For this review, take the finished solid that the model builds, in its own axes (mm). A direction names the side the tool comes from. Coordinates: 2 decimals unless noted, no trailing zeros. Loops run counter-clockwise (first coordinate to the right, second up) from the corner with the lowest first, then second, coordinate; pieces in that order, holes last. Notation, with made-up numbers: (50, 64) - (97, 64) arc R24 cw to (97, 93) - close; hole circle Ø7 at (76.25, -24.5). An arc over 180 degrees is marked (long way). One line per item, written item: value. Start each with the question number.
1. Take a section at D-D, the plane y = 1. State the section outline as (x, z) points.
2. Take a section at C-C, the plane y = -9.5. State the section outline as (x, z) points.
3. For faces 1 (the face through (-45.514, 2, 2)), 2 (the face through (-8, -35.503, 2)), 3 (the face through (-23.58, 22.1, 1.67)), list the 3-axis set-ups (+Z, -Z, +X, -X, +Y, -Y) from which the entire face can be reached by the end or side of a thin tool; tool diameter is ignored.
4. The part is to be moulded in two halves that separate along Y. For faces 4 (the face through (27.97, -32.64, 1.71)), 5 (the face through (19.195, -10.657, 1.713)), 6 (the face through (30.686, 2, 2)), say which applies: released by +Y, released by -Y, zero draft, split by the parting line, or undercut.
5. Insertion check: pin 1 (5 mm diameter, centred on x = -19.5, y = -18.5, fed in from -Z); pin 2 (1.7 mm diameter, centred on x = -62, z = 2.5, fed in from -Y); pin 3 (1 mm diameter, centred on x = -64.56, y = 37.52, fed in from -Z); pin 4 (1 mm diameter, centred on y = 7.5, z = 2.5, fed in from -X). Each pin has a flat end and moves straight along its axis. Give the tip position at first contact, or say it passes through.
6. To check wall thickness, follow line 1 (Y direction, x = 14, z = 2.8); line 2 (Y direction, x = -25, z = 1.45); line 3 (X direction, y = -8, z = 1.7). State the ranges of each line that lie inside material, in increasing order. Write a range as from..to.
7. Take a section at B-B, the plane x = -5.5. State the section outline as (y, z) points.
8. Take a section at A-A, the plane x = -22. State the section outline as (y, z) points, and give its area (3 significant figures).
```python
from build123d import *

# Parameters (mm, degrees)
F0_W        = 25.4
F0_H        = 6.35
F1_DEPTH    = 3.3782
F2_D        = 12.7
F3_D        = 19.05
F4_D        = 1.5875
F5_R        = 9.525
F6_T1_DEPTH = 28.7782
F7_R        = 5.08


# Not quite as in the source:
# - a fillet or chamfer that OpenCascade refuses, or shapes differently, is made with other operations: its cross-section is extruded or revolved along the edge and cut away or added
# - a feature names something its author has since deleted; it is built from what else it names


with BuildPart() as f1:
    # F0 (on Top) → F1 (new body)
    with BuildSketch(Plane.XY):
        Polygon((30.6859308559, 40.6974393192), (-45.5140691441, 40.6974393192), (-45.5140691441, 34.3474393192), (-45.5140691441, -35.5025606808), (30.6859308559, -35.5025606808), align=None)
        with BuildLine():
            ThreePointArc((-16.5807714399, 29.4836296191), (-15.0751376879, 29.3583825497), (-14.3562023103, 28.0295666307))
            ThreePointArc((-14.3562023103, 28.0295666307), (-14.7013947794, 27.0412204117), (-15.5868520724, 26.4826942515))
            ThreePointArc((-15.5868520724, 26.4826942515), (-23.6844276087, 22.0164519839), (-29.5755584989, 14.8881544036))
            ThreePointArc((-29.5755584989, 14.8881544036), (-31.7676732764, 14.1678257415), (-32.3633731557, 16.397036865))
            ThreePointArc((-32.3633731557, 16.397036865), (-25.8037717935, 24.5463802201), (-16.5807714399, 29.4836296191))
        make_face(mode=Mode.SUBTRACT)
        with Locations((-58.2140691441, 37.5224393192)):
            Rectangle(F0_W, F0_H)
    extrude(amount=F1_DEPTH)

    # F2 (through all)
    with Locations(Plane(origin=(0, 0, 0), x_dir=(1, 0, 0), z_dir=(0, 0, -1))):
        with Locations((-7.4140691441, -2.5974393192)):
            Hole(F2_D / 2)

    # F3 (through all)
    with Locations(Plane(origin=(0, 0, 0), x_dir=(1, 0, 0), z_dir=(0, 0, -1))):
        with Locations((11.6359308559, -21.6474393192), (11.6359308559, 16.4525606808), (-26.4640691441, 16.4525606808)):
            Hole(F3_D / 2)

    # F4 (through all)
    with Locations(Plane(origin=(0, 0, 0), x_dir=(1, 0, 0), z_dir=(0, 0, -1))):
        with Locations((-64.5640691441, -37.5224393192)):
            Hole(F4_D / 2)

    # F5
    f5_edges = [f1.edges().sort_by_distance(p)[0] for p in [
        (30.685931, -35.502561, 1.6891),
        (-45.514069, -35.502561, 1.6891),
        (30.685931, 40.697439, 1.6891),
    ]]
    fillet(f5_edges, radius=F5_R)

    # F6: fillet of radius 5.08 on 2 edges, made by hand

    # F6_s2 → F6_t1 (cut)
    with BuildSketch(Plane.XY.offset(-12.7)):
        with BuildLine():
            ThreePointArc((-70.9140691441, 35.6174393192), (-69.4261715925, 39.2095417676), (-65.8340691441, 40.6974393192))
            Line((-65.8340691441, 40.6974393192), (-70.9140691441, 40.6974393192))
            Line((-70.9140691441, 40.6974393192), (-70.9140691441, 35.6174393192))
        make_face()
        with BuildLine():
            ThreePointArc((-65.8340691441, 34.3474393192), (-69.4261715925, 35.8353368707), (-70.9140691441, 39.4274393192))
            Line((-70.9140691441, 39.4274393192), (-70.9140691441, 34.3474393192))
            Line((-70.9140691441, 34.3474393192), (-65.8340691441, 34.3474393192))
        make_face()
    extrude(amount=F6_T1_DEPTH, mode=Mode.SUBTRACT)

    # F7
    f7_edges = [f1.edges().sort_by_distance(p)[0] for p in [
        (-45.514069, 34.347439, 1.6891),
    ]]
    fillet(f7_edges, radius=F7_R)


solid = f1.part
```
Solutions:
1. outline: (-45.51, 0) - (-13.56, 0) - (-13.56, 3.38) - (-45.51, 3.38) - close; (-1.27, 0) - (30.69, 0) - (30.69, 3.38) - (-1.27, 3.38) - close
2. outline: (-45.51, 0) - (-32.97, 0) - (-32.97, 3.38) - (-45.51, 3.38) - close; (-19.95, 0) - (5.13, 0) - (5.13, 3.38) - (-19.95, 3.38) - close; (18.15, 0) - (30.69, 0) - (30.69, 3.38) - (18.15, 3.38) - close
3. face 1: +Z, -Z, -X, -Y
3. face 2: +Z, -Z, +X, -X, -Y
3. face 3: +Z, -Z
4. face 4: released by -Y
4. face 5: undercut
4. face 6: zero draft
5. pin 1: z = 0
5. pin 2: y = 34.35
5. pin 3: through
5. pin 4: x = -45.51
6. line 1: -35.5..-25.68, -7.23..12.42, 30.87..40.7
6. line 2: -35.5..-25.86, -7.04..20.84, 25.19..40.7
6. line 3: -45.51..-30.85, -22.07..7.25, 16.03..30.69
7. outline: (-35.5, 0) - (-3.46, 0) - (-3.46, 3.38) - (-35.5, 3.38) - close; (8.65, 0) - (40.7, 0) - (40.7, 3.38) - (8.65, 3.38) - close
8. outline: (-35.5, 0) - (-24.87, 0) - (-24.87, 3.38) - (-35.5, 3.38) - close; (-8.04, 0) - (23.3, 0) - (23.3, 3.38) - (-8.04, 3.38) - close; (27.17, 0) - (40.7, 0) - (40.7, 3.38) - (27.17, 3.38) - close
8. area: 187 mm2
